CAD build for the part. Positions are in the model's coordinates, mm. Face numbers are marked on the shaded views. A direction names the side the tool comes from. Give positions to 0.01 mm unless a question says otherwise; leave off trailing zeros. Order: outer loops, then holes, each group sorted by start corner. A loop starts at its lowest first (then second) coordinate and runs counter-clockwise, first axis right, second up.
Item 1: Band-saw the part on B-B on z = 18. Give the cut face in (x, y), plus the area to 3 significant figures.
Item 2: Which spindle directions (+Z, -Z, +X, -X, +Y, -Y) get a long thin tool onto all of the face, cutting with end or side? Do the marked faces 1, 2, 3 and 4. Say none if no direction does.
Item 3: Band-saw the part on C-C on y = -54.75. Give the cut face in (x, z).
Item 4: Band-saw the part on A-A on x = 94. Give the cut face in (y, z), plus the area to 3 significant figures.
Item 5: Two-plate mould, pull along X, no slides. Class the marked faces 5 and 6: released by +X, released by -X, zero draft, split by the parting line, or undercut.
Item 6: Band-saw the part on D-D on y = 0. Give the cut face in (x, z), plus the area to 3 significant figures.
Item 7: Flat gauge pins, fed straight in: P1, Ø4, axis at x = 10.5, z = 8, coming from the -Y side; P2, Ø1.5, axis at y = 11.5, z = 24, coming from the -X side; P3, Ø6, axis at y = -29.5, z = 14.5, coming from the +X side. Where does each tip first touch, or does it go through?
Item 8: Wall check: L1, parallel to Z at x = 94, y = 8.6; L2, parallel to X at y = 23, z = 10; L3, parallel to X at y = -34, z = 4.5. Give the ranges that are in metal, low to high.
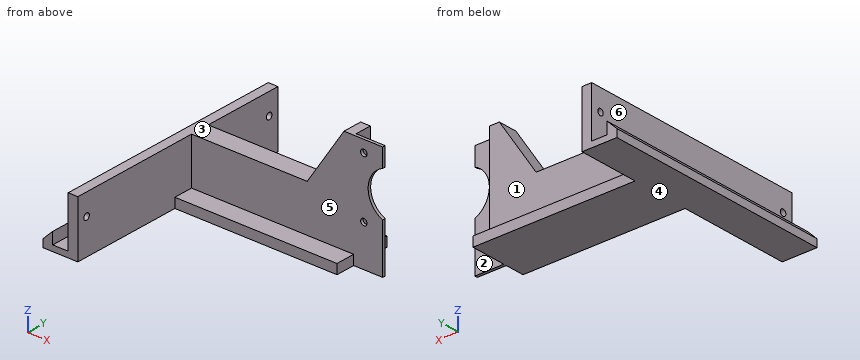
```python
from build123d import *

# Parameters (mm, degrees)
F1_R          = 1.65
F2_DEPTH      = 1.5
F3_DEPTH      = 1.5
F3_DEPTH_BACK = 8.5
F4_W          = 10
F4_H          = 5
F5_DEPTH      = 88.75
F7_DEPTH      = 60
F9_D          = 3.3


with BuildPart() as f2:
    # F1 (on offset) → F2 (new body)
    with BuildSketch(Plane.XZ.offset(-9.7)):
        with BuildLine():
            Line((88.75, 58), (88.75, 0))
            Line((88.75, 0), (103.75, 0))
            Line((103.75, 0), (103.75, 25.543561))
            ThreePointArc((103.75, 25.543561), (96.25, 37), (103.75, 48.456439))
            Line((103.75, 48.456439), (103.75, 58))
            Line((103.75, 58), (88.75, 58))
        make_face()
        with Locations((94, 21.197826)):
            Circle(F1_R, mode=Mode.SUBTRACT)
        with Locations((94, 51.947826)):
            Circle(F1_R, mode=Mode.SUBTRACT)
    extrude(amount=F2_DEPTH)

    # F1 (on offset) → F3 (join, two sides)
    with BuildSketch(Plane.XZ.offset(-9.7)) as f3_sk:
        Polygon((0, 0), (88.75, 0), (88.75, 58), (83.75, 58), (64.75, 29), (0, 29), align=None)
    extrude(amount=F3_DEPTH)
    extrude(f3_sk.sketch, amount=-F3_DEPTH_BACK)

    # F4 (on face) → F5 (join, through all)
    with BuildSketch(Plane(origin=(0, 0, 0), x_dir=(0, -1, 0), z_dir=(-1, 0, 0))):
        with Locations((-23.2, 2.5)):
            Rectangle(F4_W, F4_H)
        with Locations((-3.2, 2.5)):
            Rectangle(F4_W, F4_H)
    extrude(amount=-F5_DEPTH)

    # F6 (on Front) → F7 (join, symmetric)
    with BuildSketch(Plane.XZ):
        Polygon((-13, 4), (-13, 0), (5, 0), (5, 29), (0, 29), (0, 3), (-8, 3), (-8, 9), align=None)
    extrude(amount=F7_DEPTH, both=True)

    # F9 (through all)
    with Locations(Plane(origin=(0, 0, 0), x_dir=(0, -1, 0), z_dir=(-1, 0, 0))):
        with Locations((54.75, 18), (-54.75, 18)):
            Hole(F9_D / 2)


solid = f2.part
```
The answers:
1. outline: (0, -60) - (5, -60) - (5, -56.4) - (0, -56.4) - close; (0, -53.1) - (5, -53.1) - (5, 8.2) - (103.75, 8.2) - (103.75, 9.7) - (88.75, 9.7) - (88.75, 18.2) - (5, 18.2) - (5, 53.1) - (0, 53.1) - close; (0, 56.4) - (5, 56.4) - (5, 60) - (0, 60) - close
1. area: 1,430 mm2
2. face 1: +Z, +X, +Y
2. face 2: +Z, -Z, +X, +Y
2. face 3: +Z, -X, +Y, -Y
2. face 4: -Z, +X, -X, +Y, -Y
3. outline: (-13, 0) - (5, 0) - (5, 16.35) - (0, 16.35) - (0, 3) - (-8, 3) - (-8, 9) - (-13, 4) - close; (0, 19.65) - (5, 19.65) - (5, 29) - (0, 29) - close
4. outline: (8.2, 0) - (9.7, 0) - (9.7, 19.55) - (8.2, 19.55) - close; (8.2, 22.85) - (9.7, 22.85) - (9.7, 50.3) - (8.2, 50.3) - close; (8.2, 53.6) - (9.7, 53.6) - (9.7, 58) - (8.2, 58) - close
4. area: 77.1 mm2
5. face 5: zero draft
5. face 6: undercut
6. outline: (-13, 0) - (88.75, 0) - (88.75, 5) - (5, 5) - (5, 29) - (0, 29) - (0, 3) - (-8, 3) - (-8, 9) - (-13, 4) - close
6. area: 620 mm2
7. P1: stops at y = 8.2
7. P2: stops at x = 0
7. P3: stops at x = 5
8. L1: z = 0 to 19.55, 22.85 to 50.3, 53.6 to 58
8. L2: x = 0 to 5
8. L3: x = -12.5 to -8, 0 to 5
